```python
from build123d import *

# Parameters (mm, degrees)
BASE_FLANGE1_START = -3.175
BASE_FLANGE1_DEPTH = 3.175
EDGE_FLANGE1_DEPTH = 197.512880056


# Read off the part's stored shape, not the designer's step: Base-Flange1
# Sheet-metal steps are written as plain solids
with BuildPart() as part:
    # Base-Flange1 outline → Base-Flange1 (new body)
    with BuildSketch(Plane(origin=(0, 0, 0), x_dir=(1, 0, 0), z_dir=(0, 1, 0)).offset(BASE_FLANGE1_START)):
        Polygon((50.84064, 599.346330946), (50.84064, 396.146330946), (154.686, 291.879330946), (355.64064, 291.879330946), (355.64064, 599.346330946), align=None)
    extrude(amount=BASE_FLANGE1_DEPTH)

    # Edge-Flange1 section (across the edge) → Edge-Flange1 (add)
    with BuildSketch(Plane(origin=(248.353520056, 0, -602.521330946), x_dir=(0, 0, 1), z_dir=(-1, 0, 0))):
        with BuildLine():
            Line((-3.175, 3.175), (-3.175, 34.925))
            Line((-3.175, 34.925), (0, 34.925))
            Line((0, 34.925), (0, 3.175))
            ThreePointArc((0, 3.175), (0.92993597, 0.92993597), (3.175, 0))
            Line((3.175, 0), (3.175, -3.175))
            ThreePointArc((3.175, -3.175), (-1.315128061, -1.315128061), (-3.175, 3.175))
        make_face()
    extrude(amount=EDGE_FLANGE1_DEPTH)


solid = part.part
```
Here's how the part is built. I have some questions about the finished solid (model axes, mm). A direction names the side the tool comes from. Round coordinates to 2 decimals unless told otherwise and drop trailing zeros. Loops run counter-clockwise (first coordinate to the right, second up) from the corner with the lowest first, then second, coordinate; pieces in that order, holes last.
1. Suppose I cut it at C-C, the plane z = -518. Please give me the cut outline in (x, y) (3 decimals), and give its area (3 significant figures).
Answers:
outline: (50.841, -3.175) - (355.641, -3.175) - (355.641, 0) - (50.841, 0) - close
area: 968 mm2
2. Will these pins go through, and if not, where does the flat tip stop? pin 1 (8 mm diameter, centred on x = 95.5, z = -385, fed in from +Y); pin 2 (5 mm diameter, centred on y = 15, z = -601, fed in from +X); pin 3 (10 mm diameter, centred on x = 145, y = 3, fed in from +Z).
Answers:
pin 1: stops at y = 0
pin 2: stops at x = 248.35
pin 3: stops at z = -297.59
3. For faces 1 (the face through (201, 0, -448)), 2 (the face through (201, -3.175, -448)), which set-ups out of +Z, -Z, +X, -X, +Y, -Y let a thin tool reach every point of the face, with its end or its side?
Answers:
face 1: +Z, +X, -X, +Y
face 2: +Z, -Z, +X, -X, -Y
4. Suppose I cut it at A-A, the plane x = 213. Please give me the cut outline in (y, z) (3 decimals).
Answers:
outline: (-3.175, -599.346) arc R6.35 ccw to (3.175, -605.696) - (34.925, -605.696) - (34.925, -602.521) - (3.175, -602.521) arc R3.175 cw to (0, -599.346) - (0, -291.879) - (-3.175, -291.879) - close
5. If I drill on probe 1 along Y at (x, z) = (206, -332) (3 decimals); probe 2 along Z at (x, y) = (125, 7.5); probe 3 along Z at (x, y) = (214, 1.5), over which ranges is the centre line in solid material (lowest first)?
Answers:
probe 1: y = -3.175 to 0
probe 2: z = -605.7 to -602.52
probe 3: z = -605.47 to -602.04
6. Suppose I cut it at D-D, the plane x = 81.5. Please give me the cut outline in (y, z) (3 decimals).
Answers:
outline: (-3.175, -599.346) arc R6.35 ccw to (3.175, -605.696) - (34.925, -605.696) - (34.925, -602.521) - (3.175, -602.521) arc R3.175 cw to (0, -599.346) - (0, -365.362) - (-3.175, -365.362) - close
7. Suppose I cut it at B-B, the plane y = 18. Please give me the cut outline in (x, z), and give its area (3 significant figures).
Answers:
outline: (50.84, -605.7) - (248.35, -605.7) - (248.35, -602.52) - (50.84, -602.52) - close
area: 627 mm2
